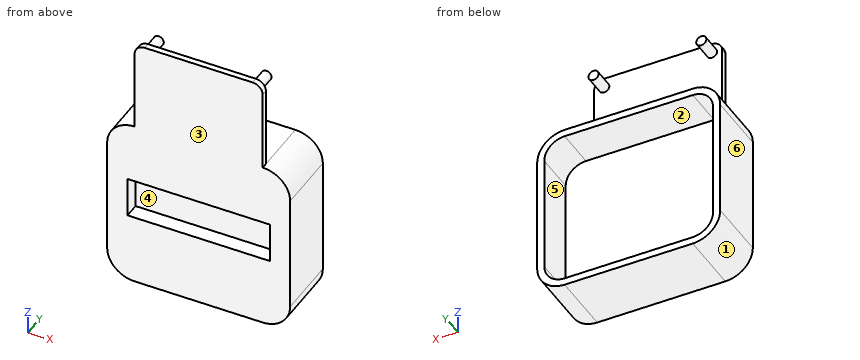
```python
from build123d import *

# Parameters (mm, degrees)
SKETCH1_W           = 90
SKETCH1_H           = 85
SKETCH1_W_2         = 70
SKETCH1_H_2         = 20
BOSS_EXTRUDE1_DEPTH = 7.5
SKETCH2_W           = 90
SKETCH2_H           = 85
BOSS_EXTRUDE2_DEPTH = 3
SKETCH3_W           = 90
SKETCH3_H           = 85
SKETCH3_W_2         = 83
SKETCH3_H_2         = 78
BOSS_EXTRUDE3_DEPTH = 20
FILLET1_R           = 10
FILLET3_R           = 10
FILLET4_R           = 10
FILLET5_R           = 10
FILLET7_R           = 13.5
FILLET8_R           = 13.5
FILLET9_R           = 13.5
FILLET10_R          = 13.5
SKETCH4_W           = 63
SKETCH4_H           = 45
BOSS_EXTRUDE4_DEPTH = 3
FILLET15_R          = 5
FILLET16_R          = 5
SKETCH7_R           = 2.5
BOSS_EXTRUDE6_DEPTH = 10


with BuildPart() as part:
    # Sketch1 → Boss-Extrude1 (new body)
    with BuildSketch(Plane(origin=(0, 0, 0), x_dir=(1, 0, 0), z_dir=(0, 1, 0))):
        with Locations((45, 42.5)):
            Rectangle(SKETCH1_W, SKETCH1_H)
        with Locations((45, 40)):
            Rectangle(SKETCH1_W_2, SKETCH1_H_2, mode=Mode.SUBTRACT)
    extrude(amount=BOSS_EXTRUDE1_DEPTH)

    # Sketch2 → Boss-Extrude2 (add)
    with BuildSketch(Plane(origin=(0, 7.5, 0), x_dir=(1, 0, 0), z_dir=(0, 1, 0))):
        with Locations((45, 42.5)):
            Rectangle(SKETCH2_W, SKETCH2_H)
    extrude(amount=BOSS_EXTRUDE2_DEPTH)

    # Sketch3 → Boss-Extrude3 (add)
    with BuildSketch(Plane(origin=(0, 10.5, 0), x_dir=(1, 0, 0), z_dir=(0, 1, 0))):
        with Locations((45, 42.5)):
            Rectangle(SKETCH3_W, SKETCH3_H)
        with Locations((45, 42.5)):
            Rectangle(SKETCH3_W_2, SKETCH3_H_2, mode=Mode.SUBTRACT)
    extrude(amount=BOSS_EXTRUDE3_DEPTH)

    # Fillet1
    fillet1_edges = [part.edges().sort_by_distance(p)[0] for p in [
        (3.5, 20.5, -81.5),
    ]]
    fillet(fillet1_edges, radius=FILLET1_R)

    # Fillet3
    fillet3_edges = [part.edges().sort_by_distance(p)[0] for p in [
        (86.5, 20.5, -81.5),
    ]]
    fillet(fillet3_edges, radius=FILLET3_R)

    # Fillet4
    fillet4_edges = [part.edges().sort_by_distance(p)[0] for p in [
        (3.5, 20.5, -3.5),
    ]]
    fillet(fillet4_edges, radius=FILLET4_R)

    # Fillet5
    fillet5_edges = [part.edges().sort_by_distance(p)[0] for p in [
        (86.5, 20.5, -3.5),
    ]]
    fillet(fillet5_edges, radius=FILLET5_R)

    # Fillet7
    fillet7_edges = [part.edges().sort_by_distance(p)[0] for p in [
        (0, 15.25, 0),
    ]]
    fillet(fillet7_edges, radius=FILLET7_R)

    # Fillet8
    fillet8_edges = [part.edges().sort_by_distance(p)[0] for p in [
        (90, 15.25, 0),
    ]]
    fillet(fillet8_edges, radius=FILLET8_R)

    # Fillet9
    fillet9_edges = [part.edges().sort_by_distance(p)[0] for p in [
        (90, 15.25, -85),
    ]]
    fillet(fillet9_edges, radius=FILLET9_R)

    # Fillet10
    fillet10_edges = [part.edges().sort_by_distance(p)[0] for p in [
        (0, 15.25, -85),
    ]]
    fillet(fillet10_edges, radius=FILLET10_R)

    # Sketch4 → Boss-Extrude4 (add)
    with BuildSketch(Plane.XZ):
        with Locations((45, 22.5)):
            Rectangle(SKETCH4_W, SKETCH4_H)
    extrude(amount=-BOSS_EXTRUDE4_DEPTH)

    # Fillet15
    fillet15_edges = [part.edges().sort_by_distance(p)[0] for p in [
        (13.5, 1.5, 45),
    ]]
    fillet(fillet15_edges, radius=FILLET15_R)

    # Fillet16
    fillet16_edges = [part.edges().sort_by_distance(p)[0] for p in [
        (76.5, 1.5, 45),
    ]]
    fillet(fillet16_edges, radius=FILLET16_R)

    # Sketch7 → Boss-Extrude6 (add)
    with BuildSketch(Plane(origin=(0, 3, 0), x_dir=(1, 0, 0), z_dir=(0, 1, 0))):
        with Locations(Location((18.5, -40, 0), (0, 0, 270))):
            Circle(SKETCH7_R)
        with Locations(Location((71.5, -40, 0), (0, 0, 270))):
            Circle(SKETCH7_R)
    extrude(amount=BOSS_EXTRUDE6_DEPTH)


solid = part.part
```
Can you work these out from the model? Positions are in its coordinate system, mm. Face numbers are marked on the shaded views. A direction names the side the tool comes from. Coordinates: 2 decimals unless noted, no trailing zeros. Order: outer loops, then holes, each group sorted by start corner. A loop starts at its lowest first (then second) coordinate and runs counter-clockwise, first axis right, second up.
1. If we section it at B-B (z = -44): Please give me the cut outline in (x, y).
2. I'm going to push flat-ended pins straight in: pin 1 (10 mm diameter, centred on x = 49.5, y = 19.5, fed in from +Z); pin 2 (5 mm diameter, centred on x = 54.5, z = -42.5, fed in from -Y); pin 3 (8 mm diameter, centred on x = 42.5, z = -61, fed in from +Y). Where does each tip first touch, or does it pass through?
3. For the marked faces 4, 5 and 6, which set-ups out of +Z, -Z, +X, -X, +Y, -Y let a thin tool reach every point of the face, with its end or its side?
4. Thinking about a two-plate mould opening in X: for the marked faces 1, 2 and 3, which applies, +X half, -X half, draft (parallel to the pull), parting line (faces both ways), or undercut?
5. If we section it at A-A (y = 25): Please give me the cut outline in (x, z), then the cut area to 3 significant figures.
6. If we section it at D-D (z = -60.5): Please give me the cut outline in (x, y), then the cut area to 4 significant figures.
7. I need wall thicknesses on line 1 (X direction, y = 4.5, z = -39); line 2 (Z direction, x = 39.5, y = 29); line 3 (Z direction, x = 24, y = 3.5). Which ranges of each line are inside material? Lowest first, please.
8. If we section it at C-C (x = 37.5): Please give me the cut outline in (y, z).
Entries:
1. outline: (0, 0) - (10, 0) - (10, 7.5) - (80, 7.5) - (80, 0) - (90, 0) - (90, 30.5) - (86.5, 30.5) - (86.5, 10.5) - (3.5, 10.5) - (3.5, 30.5) - (0, 30.5) - close
2. pin 1: stops at z = 0
2. pin 2: stops at y = 7.5
2. pin 3: stops at y = 10.5
3. face 4: -Y
3. face 5: +Y
3. face 6: +Z, -Z, -X, +Y, -Y
4. face 1: -X half
4. face 2: undercut
4. face 3: draft
5. outline: (0, -71.5) arc R13.5 ccw to (13.5, -85) - (76.5, -85) arc R13.5 ccw to (90, -71.5) - (90, -13.5) arc R13.5 ccw to (76.5, 0) - (13.5, 0) arc R13.5 ccw to (0, -13.5) - close; hole (3.5, -71.5) arc R10 ccw to (13.5, -81.5) - (76.5, -81.5) arc R10 ccw to (86.5, -71.5) - (86.5, -13.5) arc R10 ccw to (76.5, -3.5) - (13.5, -3.5) arc R10 ccw to (3.5, -13.5) - close
5. area: 1,110 mm2
6. outline: (0, 0) - (90, 0) - (90, 30.5) - (86.5, 30.5) - (86.5, 10.5) - (3.5, 10.5) - (3.5, 30.5) - (0, 30.5) - close
6. area: 1,085 mm2
7. line 1: x = 0 to 10, 80 to 90
7. line 2: z = -85 to -81.5, -3.5 to 0
7. line 3: z = -85 to -50, -30 to 0
8. outline: (0, -85) - (30.5, -85) - (30.5, -81.5) - (10.5, -81.5) - (10.5, -3.5) - (30.5, -3.5) - (30.5, 0) - (3, 0) - (3, 45) - (0, 45) - (0, -30) - (7.5, -30) - (7.5, -50) - (0, -50) - close
